```python
from build123d import *

# Parameters (mm, degrees)
F0_R     = 0.95
F0_W     = 40
F0_H     = 45
F0_W_2   = 75
F0_H_2   = 15
F0_W_3   = 64
F1_DEPTH = 4
F2_DEPTH = 8
F3_DEPTH = 10
F4_R     = 5
F5_SIZE  = 2
F6_R     = 3
F7_R     = 0.5


# Not quite as in the source:
# - a feature names something its author has since deleted; it is built from what else it names


with BuildPart() as f1:
    # F0 (on Front) → F1 (new body)
    with BuildSketch(Plane.XZ):
        with BuildLine():
            Line((0, 175), (0, 0))
            Line((0, 0), (37.5, 0))
            Line((37.5, 0), (37.5, 93.5))
            ThreePointArc((37.5, 93.5), (43, 99), (48.5, 93.5))
            Line((48.5, 93.5), (48.5, 0))
            Line((48.5, 0), (114.5, 0))
            Line((114.5, 0), (114.5, 93.5))
            ThreePointArc((114.5, 93.5), (120, 99), (125.5, 93.5))
            Line((125.5, 93.5), (125.5, 0))
            Line((125.5, 0), (191.5, 0))
            Line((191.5, 0), (191.5, 93.5))
            ThreePointArc((191.5, 93.5), (197, 99), (202.5, 93.5))
            Line((202.5, 93.5), (202.5, 0))
            Line((202.5, 0), (240, 0))
            Line((240, 0), (240, 175))
            Line((240, 175), (165, 175))
            Line((165, 175), (165, 172.5))
            Line((165, 172.5), (152, 172.5))
            Line((152, 172.5), (152, 175))
            Line((152, 175), (88, 175))
            Line((88, 175), (88, 172.5))
            Line((88, 172.5), (75, 172.5))
            Line((75, 172.5), (75, 175))
            Line((75, 175), (0, 175))
        make_face()
        with Locations((4.5, 20)):
            Circle(F0_R, mode=Mode.SUBTRACT)
        with Locations((81.5, 20)):
            Circle(F0_R, mode=Mode.SUBTRACT)
        with Locations((81.5, 55)):
            Rectangle(F0_W, F0_H, mode=Mode.SUBTRACT)
        with Locations((158.5, 20)):
            Circle(F0_R, mode=Mode.SUBTRACT)
        with Locations((235.5, 20)):
            Circle(F0_R, mode=Mode.SUBTRACT)
        with Locations((158.5, 55)):
            Rectangle(F0_W, F0_H, mode=Mode.SUBTRACT)
        with Locations((81.5, 120)):
            Rectangle(F0_W, F0_H, mode=Mode.SUBTRACT)
        with Locations((4.5, 155)):
            Circle(F0_R, mode=Mode.SUBTRACT)
        with Locations((81.5, 155)):
            Circle(F0_R, mode=Mode.SUBTRACT)
        with Locations((158.5, 120)):
            Rectangle(F0_W, F0_H, mode=Mode.SUBTRACT)
        with Locations((158.5, 155)):
            Circle(F0_R, mode=Mode.SUBTRACT)
        with Locations((235.5, 155)):
            Circle(F0_R, mode=Mode.SUBTRACT)
        with Locations((202.5, 182.5)):
            Rectangle(F0_W_2, F0_H_2)
        Polygon((165, 190), (152, 190), (152, 175), (152, 172.5), (165, 172.5), (165, 175), align=None)
        with Locations((120, 182.5)):
            Rectangle(F0_W_3, F0_H_2)
        Polygon((75, 190), (75, 175), (75, 172.5), (88, 172.5), (88, 175), (88, 190), align=None)
        with Locations((37.5, 182.5)):
            Rectangle(F0_W_2, F0_H_2)
        with BuildLine():
            Line((37.5, 93.5), (37.5, 0))
            Line((37.5, 0), (48.5, 0))
            Line((48.5, 0), (48.5, 93.5))
            ThreePointArc((48.5, 93.5), (43, 99), (37.5, 93.5))
        make_face()
        with BuildLine():
            Line((114.5, 93.5), (114.5, 0))
            Line((114.5, 0), (125.5, 0))
            Line((125.5, 0), (125.5, 93.5))
            ThreePointArc((125.5, 93.5), (120, 99), (114.5, 93.5))
        make_face()
        with BuildLine():
            Line((191.5, 93.5), (191.5, 0))
            Line((191.5, 0), (202.5, 0))
            Line((202.5, 0), (202.5, 93.5))
            ThreePointArc((202.5, 93.5), (197, 99), (191.5, 93.5))
        make_face()
    extrude(amount=F1_DEPTH)

    # F0 (on Front) → F2 (join)
    with BuildSketch(Plane.XZ):
        with BuildLine():
            Line((37.5, 93.5), (37.5, 0))
            Line((37.5, 0), (48.5, 0))
            Line((48.5, 0), (48.5, 93.5))
            ThreePointArc((48.5, 93.5), (43, 99), (37.5, 93.5))
        make_face()
        with BuildLine():
            Line((114.5, 93.5), (114.5, 0))
            Line((114.5, 0), (125.5, 0))
            Line((125.5, 0), (125.5, 93.5))
            ThreePointArc((125.5, 93.5), (120, 99), (114.5, 93.5))
        make_face()
        with BuildLine():
            Line((191.5, 93.5), (191.5, 0))
            Line((191.5, 0), (202.5, 0))
            Line((202.5, 0), (202.5, 93.5))
            ThreePointArc((202.5, 93.5), (197, 99), (191.5, 93.5))
        make_face()
    extrude(amount=F2_DEPTH)

    # F0 (on Front) → F3 (join)
    with BuildSketch(Plane.XZ):
        Polygon((75, 190), (75, 175), (75, 172.5), (88, 172.5), (88, 175), (88, 190), align=None)
        Polygon((165, 190), (152, 190), (152, 175), (152, 172.5), (165, 172.5), (165, 175), align=None)
        with Locations((202.5, 182.5)):
            Rectangle(F0_W_2, F0_H_2)
        with Locations((120, 182.5)):
            Rectangle(F0_W_3, F0_H_2)
        with Locations((37.5, 182.5)):
            Rectangle(F0_W_2, F0_H_2)
    extrude(amount=F3_DEPTH)

    # F4
    f4_edges = [f1.edges().sort_by_distance(p)[0] for p in [
        (0, -2, 0),
        (240, -2, 0),
        (138.5, -2, 32.5),
        (178.5, -2, 32.5),
        (178.5, -2, 77.5),
        (138.5, -2, 77.5),
        (138.5, -2, 142.5),
        (178.5, -2, 142.5),
        (178.5, -2, 97.5),
        (138.5, -2, 97.5),
        (61.5, -2, 32.5),
        (101.5, -2, 32.5),
        (101.5, -2, 77.5),
        (61.5, -2, 77.5),
        (101.5, -2, 97.5),
        (101.5, -2, 142.5),
        (61.5, -2, 142.5),
        (61.5, -2, 97.5),
    ]]
    fillet(f4_edges, radius=F4_R)

    # F5
    f5_edges = [f1.edges().sort_by_distance(p)[0] for p in [
        (240, -5, 190),
        (0, -5, 190),
    ]]
    chamfer(f5_edges, length=F5_SIZE)

    # F6
    f6_edges = [f1.edges().sort_by_distance(p)[0] for p in [
        (37.5, -8, 46.75),
        (43, -8, 0),
        (48.5, -8, 46.75),
        (43, -8, 99),
        (114.5, -8, 46.75),
        (120, -8, 0),
        (125.5, -8, 46.75),
        (120, -8, 99),
        (191.5, -8, 46.75),
        (197, -8, 0),
        (202.5, -8, 46.75),
        (197, -8, 99),
    ]]
    fillet(f6_edges, radius=F6_R)

    # F7
    f7_edges = [f1.edges().sort_by_distance(p)[0] for p in [
        (75, -7, 172.5),
        (75, -7, 175),
        (88, -7, 172.5),
        (88, -7, 175),
        (152, -7, 175),
        (152, -7, 172.5),
        (165, -7, 172.5),
        (165, -7, 175),
        (240, -7, 175),
        (0, -7, 175),
    ]]
    fillet(f7_edges, radius=F7_R)


solid = f1.part
```
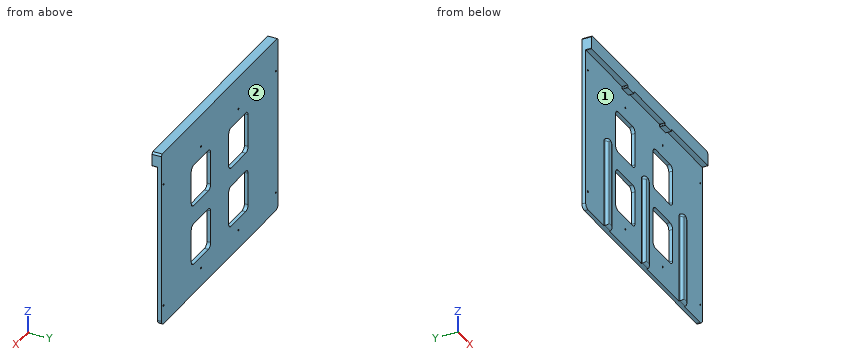
Geometry check sheet. Reference: the model listing, model coordinates, mm. Face numbers are marked on the shaded views. Round coordinates to 2 decimals unless told otherwise and drop trailing zeros. Order: outer loops, then holes, each group sorted by start corner. A loop starts at its lowest first (then second) coordinate and runs counter-clockwise, first axis right, second up. Notation, with made-up numbers: (55, -9) -> (62, -9) arc R31 ccw to (62, 26) -> close; hole circle Ø9 at (72, 39). An arc over 180 degrees is marked (long way). Return JSON: item names as keys, results as strings. Group by question number.
Q1. Section check B-B, the plane z = 13. Record the boundary of the cut face in (x, y).
Q2. Section check C-C, the plane y = -2. Count the separate pieces of the cut face and the enclosed holes in it, plus the area to 3 significant figures.
Q3. Release check for a two-part mould opening along X. For the marked faces 1 and 2 record: released by +X, released by -X, zero draft, split by the parting line, or undercut.
Q4. Gauge pin test, flat ends, axial feed: pin 1 (3 mm diameter, centred on x = 161, y = -7.5, fed in from -Z); pin 2 (0.8 mm diameter, centred on y = -4.5, z = 61.5, fed in from +X); pin 3 (0.5 mm diameter, centred on y = -4.5, z = 32.5, fed in from -X). Record the tip position at first contact, or that the pin passes through.
Q5. Section check D-D, the plane z = 164. Record the boundary of the cut face in (x, y).
Q6. Section check A-A, the plane x = 92. Record the boundary of the cut face in (y, z).
Q7. Material ranges on probe 1 along Z at (x, y) = (81.5, -1.5); probe 2 along Z at (x, y) = (235.5, -2.2); probe 3 along X at (y, z) = (-3, 155), recorded low to high. Write a range as from..to.
Numbers:
{
 "1": {"outline": "(0, -4) -> (37.5, -4) -> (37.5, -5) arc R3 ccw to (40.5, -8) -> (45.5, -8) arc R3 ccw to (48.5, -5) -> (48.5, -4) -> (114.5, -4) -> (114.5, -5) arc R3 ccw to (117.5, -8) -> (122.5, -8) arc R3 ccw to (125.5, -5) -> (125.5, -4) -> (191.5, -4) -> (191.5, -5) arc R3 ccw to (194.5, -8) -> (199.5, -8) arc R3 ccw to (202.5, -5) -> (202.5, -4) -> (240, -4) -> (240, 0) -> (0, 0) -> close"},
 "2": {"separate pieces": "1", "enclosed holes": "12", "area": "38,400 mm^2"},
 "3": {"face 1": "undercut", "face 2": "zero draft"},
 "4": {"pin 1": "z = 172.5", "pin 2": "x = 202.5", "pin 3": "x = 37.5"},
 "5": {"outline": "(0, -4) -> (240, -4) -> (240, 0) -> (0, 0) -> close"},
 "6": {"outline": "(-10, 175) -> (-4, 175) -> (-4, 142.5) -> (0, 142.5) -> (0, 190) -> (-10, 190) -> close; (-4, 0) -> (0, 0) -> (0, 32.5) -> (-4, 32.5) -> close; (-4, 77.5) -> (0, 77.5) -> (0, 97.5) -> (-4, 97.5) -> close"},
 "7": {"probe 1": "0..19.05, 20.95..32.5, 77.5..97.5, 142.5..154.05, 155.95..190", "probe 2": "0.03..19.05, 20.95..154.05, 155.95..190", "probe 3": "0..3.55, 5.45..80.55, 82.45..157.55, 159.45..234.55, 236.45..240"}
}
